```python
from build123d import *

# Parameters (mm, degrees)
F0_W      = 44.6
F0_H      = 39.1
F1_DEPTH  = 12.7
F2_R      = 1.1303
F3_DEPTH  = 25
F4_R      = 4.7625
F5_DEPTH  = 1.5
F6_R      = 0.79375
F7_DEPTH  = 11.2
F8_R      = 1.984375
F8_R_2    = 0.79375
F9_DEPTH  = 5.842
F11_DEPTH = 1.524


with BuildPart() as f1:
    # F0 (on Top) → F1 (new body)
    with BuildSketch(Plane.XY):
        with Locations((22.3, 19.55)):
            Rectangle(F0_W, F0_H)
    extrude(amount=F1_DEPTH)

    # F2 (on face) → F3 (cut)
    with BuildSketch(Plane.XY.offset(12.7)):
        with Locations((3.6, 35.5)):
            Circle(F2_R)
        with Locations((3.6, 3.6)):
            Circle(F2_R)
        with Locations((35.6, 3.6)):
            Circle(F2_R)
        with Locations((35.6, 35.5)):
            Circle(F2_R)
    extrude(amount=-F3_DEPTH, mode=Mode.SUBTRACT)

    # F4 (on face) → F5 (cut)
    with BuildSketch(Plane.XY.offset(12.7)):
        with Locations((19.3, 18.05)):
            Circle(F4_R)
    extrude(amount=-F5_DEPTH, mode=Mode.SUBTRACT)

    # F6 (on face) → F7 (cut, through all)
    with BuildSketch(Plane.XY.offset(11.2)):
        with Locations((19.3, 18.05)):
            Circle(F6_R)
    extrude(amount=-F7_DEPTH, mode=Mode.SUBTRACT)

    # F8 (on face) → F9 (cut)
    with BuildSketch(Plane(origin=(0, 0, 0), x_dir=(1, 0, 0), z_dir=(0, 0, -1))):
        with Locations((19.3, -18.05)):
            Circle(F8_R)
        with Locations((19.3, -18.05)):
            Circle(F8_R_2, mode=Mode.SUBTRACT)
    extrude(amount=-F9_DEPTH, mode=Mode.SUBTRACT)

    # F10 (on face) → F11 (cut)
    with BuildSketch(Plane.XY.offset(12.7)):
        with BuildLine():
            ThreePointArc((19.939, 13.3305630368), (19.3040360368, 13.2875017102), (18.669, 13.3294867599))
            Line((18.669, 13.3294867599), (18.669, 0))
            Line((18.669, 0), (19.939, 0))
            Line((19.939, 0), (19.939, 13.3305630368))
        make_face()
    extrude(amount=-F11_DEPTH, mode=Mode.SUBTRACT)


solid = f1.part
```
Geometry check sheet. Reference: the model listing, model coordinates, mm. A direction names the side the tool comes from. Give positions to 0.01 mm unless a question says otherwise; leave off trailing zeros. Order: outer loops, then holes, each group sorted by start corner. A loop starts at its lowest first (then second) coordinate and runs counter-clockwise, first axis right, second up.
1. Section check C-C, the plane y = 35.5. Enter the section's corners in (x, z).
2. Access from +Z, -Z, +X, -X, +Y, -Y to the whole of each face (thin tool, end or side, straight path). Record for faces 1 (the face through (0, 19, 6)), 2 (the face through (19.939, 7, 12)), 3 (the face through (19, 19, 5.842)), 4 (the face through (20.3, 18.1, 11.2)).
3. Gauge pin test, flat ends, axial feed: pin 1 Ø3 at (x, z) = (33, 10) entering from -Y; pin 2 Ø2.5 at (x, y) = (19.3, 18.05) entering from -Z; pin 3 Ø1.3 at (x, y) = (19.3, 18.05) entering from -Z; pin 4 Ø3 at (x, y) = (21, 20) entering from +Z. Record the tip position at first contact, or that the pin passes through.
4. Section check B-B, the plane x = 35.6. Enter the section's corners in (y, z), and give its area (3 significant figures).
5. Thickness scan on L1, parallel to Y at x = 3.6, z = 7.5; L2, parallel to X at y = 4, z = 1.25; L3, parallel to Y at x = 19.3, z = 9.3. Record the ranges inside material, lowest first.
6. Release check for a two-part mould opening along Y. For faces 5 (the face through (18.669, 7, 12)), 6 (the face through (36.644, 3.167, 6.439)), 7 (the face through (4.122, 2.597, 6.439)), 8 (the face through (22, 39.1, 6)) record: pulls with the +Y half, pulls with the -Y half, needs draft (parallel to the pull), parting line crosses it, or undercut.
7. Section check D-D, the plane z = 2.75. Enter the section's corners in (x, y).
Values follow:
1. outline: (0, 0) - (2.47, 0) - (2.47, 12.7) - (0, 12.7) - close; (4.73, 0) - (34.47, 0) - (34.47, 12.7) - (4.73, 12.7) - close; (36.73, 0) - (44.6, 0) - (44.6, 12.7) - (36.73, 12.7) - close
2. face 1: +Z, -Z, -X, +Y, -Y
2. face 2: +Z, -Y
2. face 3: -Z
2. face 4: +Z
3. pin 1: stops at y = 0
3. pin 2: stops at z = 5.84
3. pin 3: passes through
3. pin 4: stops at z = 11.2
4. outline: (0, 0) - (2.47, 0) - (2.47, 12.7) - (0, 12.7) - close; (4.73, 0) - (34.37, 0) - (34.37, 12.7) - (4.73, 12.7) - close; (36.63, 0) - (39.1, 0) - (39.1, 12.7) - (36.63, 12.7) - close
4. area: 439 mm2
5. L1: y = 0 to 2.47, 4.73 to 34.37, 36.63 to 39.1
5. L2: x = 0 to 2.54, 4.66 to 34.54, 36.66 to 44.6
5. L3: y = 0 to 17.26, 18.84 to 39.1
6. face 5: needs draft
6. face 6: undercut
6. face 7: undercut
6. face 8: pulls with the +Y half
7. outline: (0, 0) - (44.6, 0) - (44.6, 39.1) - (0, 39.1) - close; hole circle Ø2.26 at (3.6, 3.6); hole circle Ø2.26 at (3.6, 35.5); hole circle Ø3.97 at (19.3, 18.05); hole circle Ø2.26 at (35.6, 3.6); hole circle Ø2.26 at (35.6, 35.5)
